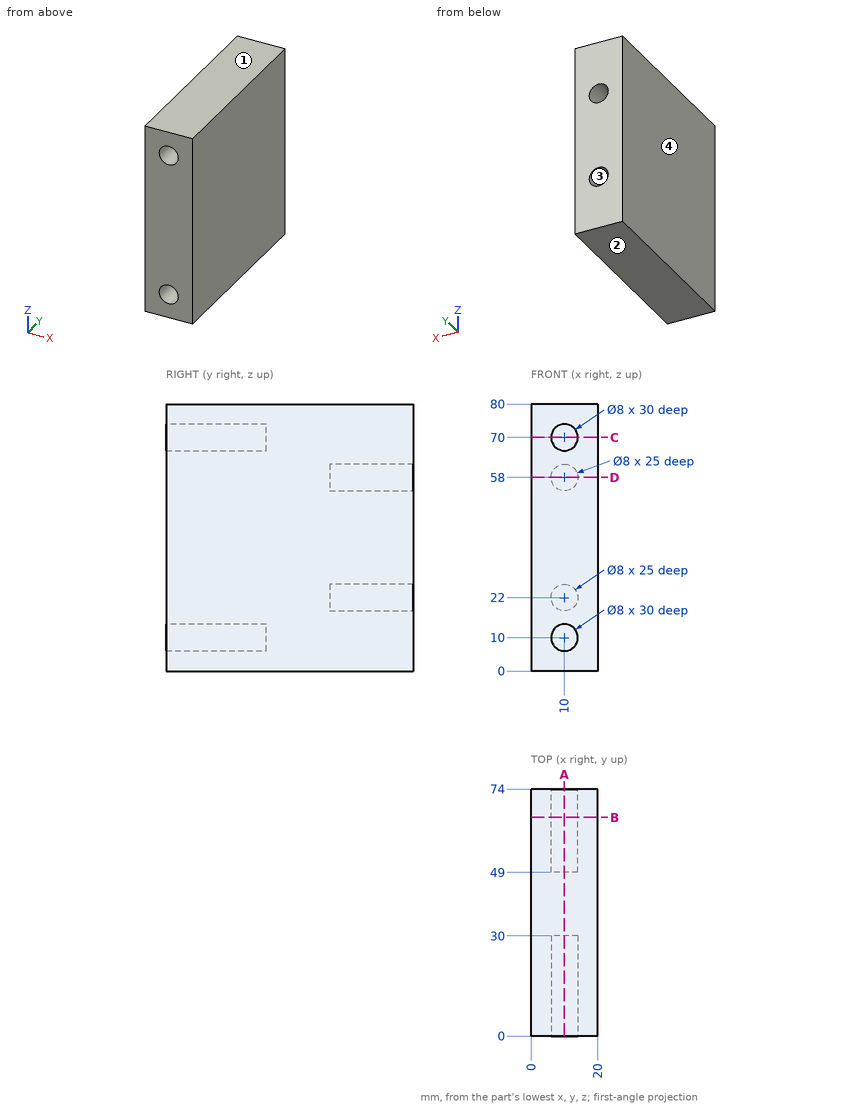
Geometry check sheet. Reference: drawing and pictorial views, mm from the part's lowest x, y, z. Round coordinates to 2 decimals unless told otherwise and drop trailing zeros. Loops run counter-clockwise (first coordinate to the right, second up) from the corner with the lowest first, then second, coordinate; pieces in that order, holes last. Notation, with made-up numbers: (36, -2) -> (74, -2) arc R6 cw to (74, 2) -> close; hole circle Ø3 at (40.25, 39). An arc over 180 degrees is marked (long way). Use a Markdown table: item, result.
(1) Sectioned sample at B-B (y = 65.5). Enter the section's corners in (x, z).
Calculated:
| item | result |
|---|---|
| outline | (0, 0) -> (20, 0) -> (20, 80) -> (0, 80) -> close; hole circle Ø8 at (10, 22); hole circle Ø8 at (10, 58) |
(2) Mould release check, pull along Z, two halves, no side actions. Record for the marked faces 1, 2, 3 and 4: released by +Z, released by -Z, zero draft, split by the parting line, or undercut.
Calculated:
| item | result |
|---|---|
| face 1 | released by +Z |
| face 2 | released by -Z |
| face 3 | undercut |
| face 4 | zero draft |
(3) Sectioned sample at C-C (z = 70). Enter the section's corners in (x, y).
Calculated:
| item | result |
|---|---|
| outline | (0, 0) -> (6, 0) -> (6, 30) -> (14, 30) -> (14, 0) -> (20, 0) -> (20, 74) -> (0, 74) -> close |
(4) Go/stop test with flat-tipped pins: P1, Ø4, axis at x = 10, z = 21.5, coming from the +Y side; P2, Ø10.5, axis at x = 10, z = 58, coming from the +Y side; P3, Ø5, axis at x = 10, z = 70, coming from the -Y side. Record where each tip stops, or that it passes through.
Calculated:
| item | result |
|---|---|
| P1 | y = 49 |
| P2 | y = 74 |
| P3 | y = 30 |
(5) Scan lines: probe 1 along X at (y, z) = (12, 70); probe 2 along Z at (x, y) = (7.5, 29.5); probe 3 along Z at (x, y) = (11.25, 59.5). Record each from-to range of solid material in increasing order.
Calculated:
| item | result |
|---|---|
| probe 1 | 0 to 6, 14 to 20 |
| probe 2 | 0 to 6.88, 13.12 to 66.88, 73.12 to 80 |
| probe 3 | 0 to 18.2, 25.8 to 54.2, 61.8 to 80 |
(6) Sectioned sample at A-A (x = 10). Enter the section's corners in (y, z).
Calculated:
| item | result |
|---|---|
| outline | (0, 0) -> (74, 0) -> (74, 18) -> (49, 18) -> (49, 26) -> (74, 26) -> (74, 54) -> (49, 54) -> (49, 62) -> (74, 62) -> (74, 80) -> (0, 80) -> (0, 74) -> (30, 74) -> (30, 66) -> (0, 66) -> (0, 14) -> (30, 14) -> (30, 6) -> (0, 6) -> close |
(7) Sectioned sample at D-D (z = 58). Enter the section's corners in (x, y).
Calculated:
| item | result |
|---|---|
| outline | (0, 0) -> (20, 0) -> (20, 74) -> (14, 74) -> (14, 49) -> (6, 49) -> (6, 74) -> (0, 74) -> close |
